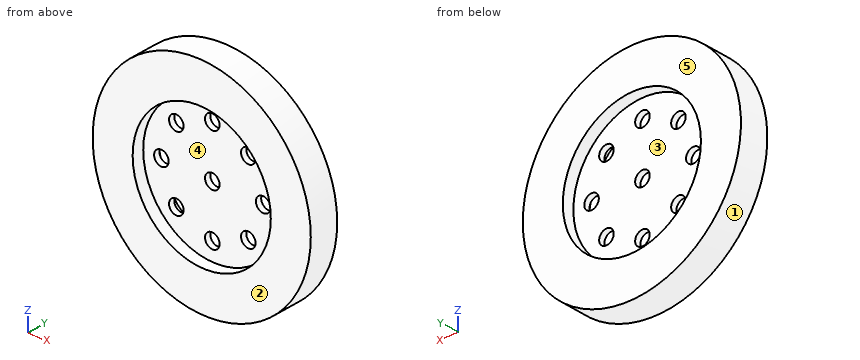
from build123d import *

# Parameters (mm, degrees)
SKETCH1_R           = 75
SKETCH1_R_2         = 43
BOSS_EXTRUDE1_DEPTH = 20
SKETCH2_R           = 43
BOSS_EXTRUDE2_DEPTH = 20
SKETCH3_R           = 47.5
CUT_EXTRUDE1_DEPTH  = 8
SKETCH6_R           = 5
CUT_EXTRUDE4_DEPTH  = 13
SKETCH4_R           = 47.5
CUT_EXTRUDE2_DEPTH  = 8
SKETCH5_R           = 3
SKETCH5_R_2         = 5
CUT_EXTRUDE3_DEPTH  = 13


with BuildPart() as part:
    # Sketch1 → Boss-Extrude1 (new body)
    with BuildSketch(Plane(origin=(0, 0, 0), x_dir=(1, 0, 0), z_dir=(0, 1, 0))):
        Circle(SKETCH1_R)
        Circle(SKETCH1_R_2, mode=Mode.SUBTRACT)
    extrude(amount=BOSS_EXTRUDE1_DEPTH)

    # Sketch2 → Boss-Extrude2 (add)
    with BuildSketch(Plane(origin=(0, 20, 0), x_dir=(1, 0, 0), z_dir=(0, 1, 0))):
        Circle(SKETCH2_R)
    extrude(amount=-BOSS_EXTRUDE2_DEPTH)

    # Sketch3 → Cut-Extrude1 (cut)
    with BuildSketch(Plane(origin=(0, 20, 0), x_dir=(1, 0, 0), z_dir=(0, 1, 0))):
        Circle(SKETCH3_R)
    extrude(amount=-CUT_EXTRUDE1_DEPTH, mode=Mode.SUBTRACT)

    # Sketch6 → Cut-Extrude4 (cut, through all)
    with BuildSketch(Plane(origin=(0, 12, 0), x_dir=(1, 0, 0), z_dir=(0, 1, 0))):
        Circle(SKETCH6_R)
    extrude(amount=-CUT_EXTRUDE4_DEPTH, mode=Mode.SUBTRACT)

    # Sketch4 → Cut-Extrude2 (cut)
    with BuildSketch(Plane.XZ):
        Circle(SKETCH4_R)
    extrude(amount=-CUT_EXTRUDE2_DEPTH, mode=Mode.SUBTRACT)

    # Sketch5 → Cut-Extrude3 (cut, through all)
    with BuildSketch(Plane(origin=(0, 12, 0), x_dir=(1, 0, 0), z_dir=(0, 1, 0))):
        Circle(SKETCH5_R)
        with Locations((0, 35)):
            Circle(SKETCH5_R_2)
        with Locations((24.748737342, 24.748737342)):
            Circle(SKETCH5_R_2)
        with Locations((35, 0)):
            Circle(SKETCH5_R_2)
        with Locations((24.748737342, -24.748737342)):
            Circle(SKETCH5_R_2)
        with Locations((0, -35)):
            Circle(SKETCH5_R_2)
        with Locations((-24.748737342, -24.748737342)):
            Circle(SKETCH5_R_2)
        with Locations((-35, 0)):
            Circle(SKETCH5_R_2)
        with Locations((-24.748737342, 24.748737342)):
            Circle(SKETCH5_R_2)
    extrude(amount=-CUT_EXTRUDE3_DEPTH, mode=Mode.SUBTRACT)


solid = part.part
Verification items for the finished model (mm, model axes). Face numbers are marked on the shaded views. A direction names the side the tool comes from. Coordinates: 2 decimals unless noted, no trailing zeros. Write each loop counter-clockwise with the first axis right and the second up, starting at its lowest first coordinate (ties: lowest second). Pieces come first, ordered by that corner, then holes. Notation, with made-up numbers: M 49,43 L 61,43 A11 cw 61,50 Z; hole C 18.25,4 d1. An arc over 180 degrees is marked long. One line per question, with ' | ' between items.
1) Access from +Z, -Z, +X, -X, +Y, -Y to the whole of each face (thin tool, end or side, straight path). Record for the marked faces 4 and 5.
Solutions:
face 4: -Y | face 5: +Z, -Z, +X, -X, +Y
2) Sectioned sample at A-A on z = 0. Record the cut outline in (x, y), then the cut area to 3 significant figures.
Solutions:
outline: M -75,0 L -47.5,0 L -47.5,8 L -40,8 L -40,12 L -47.5,12 L -47.5,20 L -75,20 Z; M -30,8 L -5,8 L -5,12 L -30,12 Z; M 5,8 L 30,8 L 30,12 L 5,12 Z; M 40,8 L 47.5,8 L 47.5,0 L 75,0 L 75,20 L 47.5,20 L 47.5,12 L 40,12 Z | area: 1,360 mm^2
3) Material ranges on L1, parallel to Z at x = 0, y = 9.05; L2, parallel to Z at x = 0, y = 3, recorded low to high.
Solutions:
L1: -75 to -40, -30 to -5, 5 to 30, 40 to 75 | L2: -75 to -47.5, 47.5 to 75
4) Sectioned sample at D-D on x = 0. Record the cut outline in (y, z), then the cut area to 3 significant figures.
Solutions:
outline: M 0,-75 L 20,-75 L 20,-47.5 L 12,-47.5 L 12,-40 L 8,-40 L 8,-47.5 L 0,-47.5 Z; M 0,47.5 L 8,47.5 L 8,40 L 12,40 L 12,47.5 L 20,47.5 L 20,75 L 0,75 Z; M 8,-30 L 12,-30 L 12,-5 L 8,-5 Z; M 8,5 L 12,5 L 12,30 L 8,30 Z | area: 1,360 mm^2
5) Sectioned sample at B-B on x = -35. Record the cut outline in (y, z), then the cut area to 3 significant figures.
Solutions:
outline: M 0,-66.33 L 20,-66.33 L 20,-32.11 L 12,-32.11 L 12,-5 L 8,-5 L 8,-32.11 L 0,-32.11 Z; M 0,32.11 L 8,32.11 L 8,5 L 12,5 L 12,32.11 L 20,32.11 L 20,66.33 L 0,66.33 Z | area: 1,590 mm^2
6) Release check for a two-part mould opening along X. For the marked faces 1, 2 and 3 record: +X half, -X half, draft (parallel to the pull), parting line (faces both ways), or undercut.
Solutions:
face 1: parting line | face 2: draft | face 3: undercut
7) Depth check by flat-ended pin: pin 1 Ø13 at (x, z) = (-24.75, -24.75) entering from +Y; pin 2 Ø13 at (x, z) = (0, 0) entering from -Y; pin 3 Ø12 at (y, z) = (11.5, -36.5) entering from +X. Enter the tip coordinate at first touch or a pass-through.
Solutions:
pin 1: y = 12 | pin 2: y = 8 | pin 3: x = 68.52
8) Sectioned sample at C-C on z = 35. Record the cut outline in (x, y).
Solutions:
outline: M -66.33,0 L -32.11,0 L -32.11,8 L -5,8 L -5,12 L -32.11,12 L -32.11,20 L -66.33,20 Z; M 5,8 L 32.11,8 L 32.11,0 L 66.33,0 L 66.33,20 L 32.11,20 L 32.11,12 L 5,12 Z
